Geometry: see drawing. Coordinates: mm, zero at the bounding-box minimum. Round coordinates to 2 decimals unless told otherwise and drop trailing zeros. Loops run counter-clockwise (first coordinate to the right, second up) from the corner with the lowest first, then second, coordinate; pieces in that order, holes last. Notation, with made-up numbers: (0, 39) - (43, 39) arc R19 ccw to (43, 69) - close; hole circle Ø3 at (-33.75, 29.25). An arc over 180 degrees is marked (long way). Use CSV: the item, a comma, the result in double quotes.
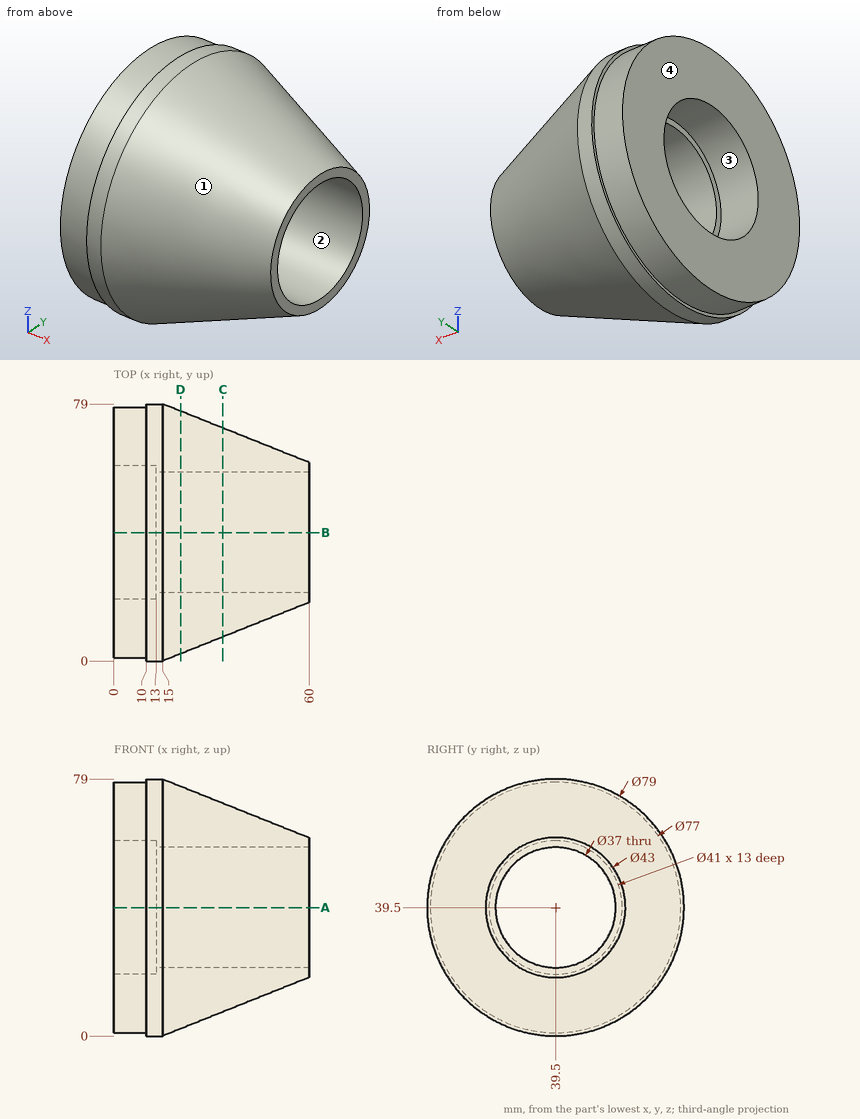
Item 1: Pin query (flat end, axial travel): P1, Ø3, axis at y = 59.5, z = 54, coming from the +X side; P2, Ø8, axis at x = 31.5, z = 17.5, coming from the -Y side; P3, Ø1.5, axis at x = 7.5, z = 64.5, coming from the +Y side; P4, Ø23.5, axis at y = 20, z = 22, coming from the -X side. Return the tip coordinate at first contact, or that it passes through.
Final values:
P1,"stops at x = 55.74"
P2,"stops at y = 11.34"
P3,"stops at y = 69.4"
P4,"stops at x = 0"
Item 2: Mould query, pull axis Z, two halves, no side actions, for the marked faces 1, 2, 3 and 4. Classes: released by +Z, released by -Z, zero draft, split by the parting line, or undercut.
Final values:
face 1,"split by the parting line"
face 2,"undercut"
face 3,"undercut"
face 4,"zero draft"
Item 3: Section D-D on x = 20.5. Return the cut outline in (y, z), plus the area to 3 significant figures.
Final values:
outline,"circle Ø74.6 at (39.5, 39.5); hole circle Ø37 at (39.5, 39.5)"
area,"3,300 mm²"
Item 4: Section A-A on z = 39.5. Return the cut outline in (x, y).
Final values:
outline,"(0, 1) - (10, 1) - (10, 0) - (15, 0) - (60, 18) - (60, 21) - (13, 21) - (13, 19) - (0, 19) - close; (0, 60) - (13, 60) - (13, 58) - (60, 58) - (60, 61) - (15, 79) - (10, 79) - (10, 78) - (0, 78) - close"
Item 5: Material intervals for line 1 (Y direction, x = 5.75, z = 39.5); line 2 (Z direction, x = 6.5, y = 28); line 3 (Y direction, x = 48, z = 23), sorted ascending.
Final values:
line 1,"y = 1 to 19, 60 to 78"
line 2,"z = 2.76 to 22.53, 56.47 to 76.24"
line 3,"y = 19.02 to 31.13, 47.87 to 59.98"
Item 6: Section C-C on x = 33.5. Return the cut outline in (y, z), plus the area to 3 significant figures.
Final values:
outline,"circle Ø64.2 at (39.5, 39.5); hole circle Ø37 at (39.5, 39.5)"
area,"2,160 mm²"
